Can you work these out from the model? Positions are in its coordinate system, mm. Coordinates: 2 decimals unless noted, no trailing zeros. Loops run counter-clockwise (first coordinate to the right, second up) from the corner with the lowest first, then second, coordinate; pieces in that order, holes last.
```python
from build123d import *

# Parameters (mm, degrees)
F0_W     = 88.9
F0_H     = 12.7
F1_DEPTH = 96.6975968
F3_D     = 5.1054
F3_DEPTH = 13.97
F3_TIP   = 1.5338169022
F5_D     = 5.1054
F5_DEPTH = 13.97
F5_TIP   = 1.5338169022


with BuildPart() as f1:
    # F0 (on Top) → F1 (new body)
    with BuildSketch(Plane.XY):
        with Locations((-44.45, 6.35)):
            Rectangle(F0_W, F0_H)
    extrude(amount=F1_DEPTH)

    # F3
    with Locations(Plane.XY.offset(96.6975968)):
        with Locations((-76.2, 6.35), (-12.7, 6.35)):
            Hole(F3_D / 2, depth=F3_DEPTH)
            with Locations((0, 0, -(F3_DEPTH + F3_TIP / 2))):  # 118° drill point
                Cone(0, F3_D / 2, F3_TIP, mode=Mode.SUBTRACT)

    # F5
    with Locations(Plane(origin=(0, 0, 0), x_dir=(1, 0, 0), z_dir=(0, 0, -1))):
        with Locations((-76.2, -6.35), (-12.7, -6.35)):
            Hole(F5_D / 2, depth=F5_DEPTH)
            with Locations((0, 0, -(F5_DEPTH + F5_TIP / 2))):  # 118° drill point
                Cone(0, F5_D / 2, F5_TIP, mode=Mode.SUBTRACT)


solid = f1.part
```
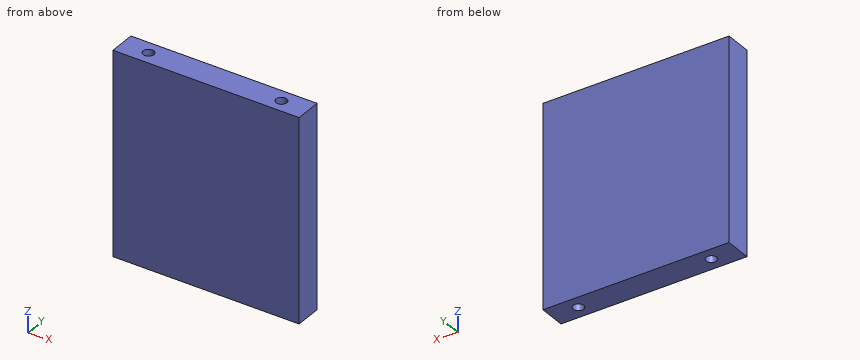
(1) If I drill on probe 1 along X at (y, z) = (6.35, 87.5); probe 2 along Y at (x, z) = (-12.7, 90.25), over which ranges is the centre line in solid material (lowest first)?
Check values:
probe 1: x = -88.9 to -78.75, -73.65 to -15.25, -10.15 to 0
probe 2: y = 0 to 3.8, 8.9 to 12.7
(2) I'm going to push a flat-ended pin straight in: pin 1 (4 mm diameter, centred on x = -76.2, y = 6.35, fed in from +Z). Where does the tip first touch, or does it pass through?
Check values:
pin 1: stops at z = 82.4
(3) I want a section at A-A on z = 86. Write out the boundary of the cut face in (x, y), then the cut area to 3 significant figures.
Check values:
outline: (-88.9, 0) - (0, 0) - (0, 12.7) - (-88.9, 12.7) - close; hole circle Ø5.11 at (-76.2, 6.35); hole circle Ø5.11 at (-12.7, 6.35)
area: 1,090 mm2
